Work out the finished part from the listing and answer in its coordinate system (mm). A direction names the side the tool comes from. Round coordinates to 2 decimals unless told otherwise and drop trailing zeros. Write each loop counter-clockwise with the first axis right and the second up, starting at its lowest first coordinate (ties: lowest second). Pieces come first, ordered by that corner, then holes. Notation, with made-up numbers: (45, 68) - (56, 68) arc R10 ccw to (56, 87) - close; hole circle Ø11 at (-3, -22.5). An arc over 180 degrees is marked (long way). Answer as a JSON object with one key per item and string values.
```python
from build123d import *

# Parameters (mm, degrees)
F0_R           = 35
F1_DEPTH       = 15
F2_R           = 25
F3_DEPTH       = 2.6
F4_R           = 18
F5_DEPTH       = 5
F6_D           = 5
F7_D           = 6.5
F7_CSINK_D     = 12.6
F7_CSINK_ANGLE = 90
F8_D           = 16


with BuildPart() as f1:
    # F0 (on Top) → F1 (new body)
    with BuildSketch(Plane.XY):
        Circle(F0_R)
    extrude(amount=F1_DEPTH)

    # F2 (on face) → F3 (cut)
    with BuildSketch(Plane.XY.offset(15)):
        Circle(F2_R)
    extrude(amount=-F3_DEPTH, mode=Mode.SUBTRACT)

    # F4 (on face) → F5 (cut)
    with BuildSketch(Plane(origin=(0, 0, 0), x_dir=(1, 0, 0), z_dir=(0, 0, -1))):
        Circle(F4_R)
    extrude(amount=-F5_DEPTH, mode=Mode.SUBTRACT)

    # F6 (through all)
    with Locations(Plane(origin=(0, 0, 0), x_dir=(1, 0, 0), z_dir=(0, 0, -1))):
        with Locations((-6.6152965396, -23.0702807025), (-16.671800891, 17.2641552081), (23.2870974306, 5.8061254944)):
            Hole(F6_D / 2)

    # F7 (through all)
    with Locations(Plane(origin=(0, 0, 0), x_dir=(1, 0, 0), z_dir=(0, 0, -1))):
        with Locations((30, 0), (-30, 0), (0, -29.25), (0, 29.25)):
            CounterSinkHole(F7_D / 2, F7_CSINK_D / 2, counter_sink_angle=F7_CSINK_ANGLE)

    # F8 (through all)
    with Locations(Plane(origin=(0, 0, 0), x_dir=(1, 0, 0), z_dir=(0, 0, -1))):
        with Locations((0, 0)):
            Hole(F8_D / 2)


solid = f1.part
```
Item 1: A cutting plane is placed at A-A (y = 0). Write down the section's boundary in (x, z).
Results found:
{"outline": "(-35, 1.3) - (-33.25, 3.05) - (-33.25, 15) - (-35, 15) - close; (-26.75, 3.05) - (-23.7, 0) - (-18, 0) - (-18, 5) - (-8, 5) - (-8, 12.4) - (-25, 12.4) - (-25, 15) - (-26.75, 15) - close; (8, 5) - (18, 5) - (18, 0) - (23.7, 0) - (26.75, 3.05) - (26.75, 15) - (25, 15) - (25, 12.4) - (8, 12.4) - close; (33.25, 3.05) - (35, 1.3) - (35, 15) - (33.25, 15) - close"}
Item 2: Determine the mould class of faces 1 (the cylindrical face through (32.33, -13.41, 7.39)), 2 (the flat face through (23.2, -10.2, 15)), 3 (the flat face through (8, 4, 5)) for opening direction X: pulls with the +X half, pulls with the -X half, needs draft (parallel to the pull), parting line crosses it, or undercut.
Results found:
{"face 1": "parting line crosses it", "face 2": "needs draft", "face 3": "undercut"}
Item 3: A cutting plane is placed at B-B (x = 0). Write down the section's boundary in (y, z).
Results found:
{"outline": "(-35, 0.55) - (-32.5, 3.05) - (-32.5, 15) - (-35, 15) - close; (-26, 3.05) - (-22.95, 0) - (-18, 0) - (-18, 5) - (-8, 5) - (-8, 12.4) - (-25, 12.4) - (-25, 15) - (-26, 15) - close; (8, 5) - (18, 5) - (18, 0) - (22.95, 0) - (26, 3.05) - (26, 15) - (25, 15) - (25, 12.4) - (8, 12.4) - close; (32.5, 3.05) - (35, 0.55) - (35, 15) - (32.5, 15) - close"}
Item 4: For faces 4 (the cylindrical face through (7, -24, 14)), 5 (the cylindrical face through (-2.343, -17.847, 2.465)), 6 (the flat face through (15, -15, 0)), determine the directions among +Z, -Z, +X, -X, +Y, -Y from which every point of the face is accessible in a straight line to the end or side of a thin tool.
Results found:
{"face 4": "+Z", "face 5": "-Z", "face 6": "-Z, +X, -X, +Y, -Y"}
Item 5: A cutting plane is placed at D-D (y = -29.25). Write down the section's boundary in (x, z).
Results found:
{"outline": "(-19.22, 0) - (-6.3, 0) - (-3.25, 3.05) - (-3.25, 15) - (-19.22, 15) - close; (3.25, 3.05) - (6.3, 0) - (19.22, 0) - (19.22, 15) - (3.25, 15) - close"}
Item 6: Consider line 1 along Y through (x, z) = (0, 6.75); line 2 along Y through (x, z) = (-4.5, 9); line 3 along X through (y, z) = (-15.5, 4.25). Determine where each line is inside the solid, lowest interval first.
Results found:
{"line 1": "-35 to -32.5, -26 to -8, 8 to 26, 32.5 to 35", "line 2": "-34.71 to -6.61, 6.61 to 21.74, 24.4 to 34.71", "line 3": "-31.38 to -18.44, -14.9 to -9.15, 9.15 to 31.38"}
Item 7: Each of these flat-tipped pins is pushed along its axis until it touches: P1, Ø6, axis at y = 16.5, z = 2, coming from the -X side; P2, Ø7.5, axis at x = -30, y = 0, coming from the +Z side; P3, Ø1, axis at x = -12.5, z = 10, coming from the -Y side; P4, Ø8, axis at y = -26, z = 13.5, coming from the -X side. Where does it stop, or does it pass through?
Results found:
{"P1": "x = -32.29", "P2": "z = 15", "P3": "y = -32.88", "P4": "x = -27.22"}
Item 8: A cutting plane is placed at C-C (z = 10). Give the number of separate pieces and of enclosed holes in the cut face, and give its area (3 significant figures).
Results found:
{"separate pieces": "1", "enclosed holes": "8", "area": "3,460 mm²"}
